```python
from build123d import *

# Parameters (mm, degrees)
SKETCH1_R           = 10
BOSS_EXTRUDE1_DEPTH = 15.1
SKETCH2_R           = 8.25
CUT_EXTRUDE1_DEPTH  = 7
SKETCH3_R           = 6.35
CUT_EXTRUDE2_DEPTH  = 8.1
SKETCH7_R           = 10
BOSS_EXTRUDE2_DEPTH = 10
BOSS_EXTRUDE2_TAPER = 27
SKETCH8_R           = 5.5
CUT_EXTRUDE3_DEPTH  = 10


with BuildPart() as part:
    # Sketch1 → Boss-Extrude1 (new body)
    with BuildSketch(Plane(origin=(0, 0, 0), x_dir=(1, 0, 0), z_dir=(0, 1, 0))):
        with Locations(Location((0, 0, 0), (0, 0, 270))):
            Circle(SKETCH1_R)
    extrude(amount=BOSS_EXTRUDE1_DEPTH)

    # Sketch2 → Cut-Extrude1 (cut)
    with BuildSketch(Plane(origin=(0, 0, 0), x_dir=(-1, 0, 0), z_dir=(0, -1, 0))):
        with Locations(Location((0, 0, 0), (0, 0, 90))):
            Circle(SKETCH2_R)
    extrude(amount=-CUT_EXTRUDE1_DEPTH, mode=Mode.SUBTRACT)

    # Sketch3 → Cut-Extrude2 (cut)
    with BuildSketch(Plane.XZ.offset(-7)):
        with Locations(Location((0, 0, 0), (0, 0, 270))):
            Circle(SKETCH3_R)
    extrude(amount=-CUT_EXTRUDE2_DEPTH, mode=Mode.SUBTRACT)

    # Sketch7 → Boss-Extrude2 (add)
    with BuildSketch(Plane(origin=(0, 15.1, 0), x_dir=(1, 0, 0), z_dir=(0, 1, 0))):
        with Locations(Location((0, 0, 0), (0, 0, 270))):
            Circle(SKETCH7_R)
    extrude(amount=BOSS_EXTRUDE2_DEPTH, taper=BOSS_EXTRUDE2_TAPER)

    # Sketch8 → Cut-Extrude3 (cut)
    with BuildSketch(Plane(origin=(0, 25.1, 0), x_dir=(1, 0, 0), z_dir=(0, 1, 0))):
        with Locations(Location((0, 0, 0), (0, 0, 270))):
            Circle(SKETCH8_R)
    extrude(amount=-CUT_EXTRUDE3_DEPTH, mode=Mode.SUBTRACT)

    # Sketch9 → Cut-Revolve1 (revolve, cut)
    with BuildSketch(Plane.XY, mode=Mode.PRIVATE) as cut_revolve1_sk:
        Polygon((10, 0), (10, 7.55), (9, 0), align=None)
    revolve(cut_revolve1_sk.sketch.rotate(Axis((0, -5.35411367, 0), (0, 1, 0)), 90), axis=Axis((0, -5.35411367, 0), (0, 1, 0)), mode=Mode.SUBTRACT)


solid = part.part
```
Geometry: final body of the model. Coordinates: model frame, mm. A direction names the side the tool comes from. Round coordinates to 2 decimals unless told otherwise and drop trailing zeros. Loops run counter-clockwise (first coordinate to the right, second up) from the corner with the lowest first, then second, coordinate; pieces in that order, holes last. Notation, with made-up numbers: (70.25, 34.25) -> (115.25, 34.25) arc R20 cw to (115.25, 68.25) -> close; hole circle Ø3 at (66, 22). An arc over 180 degrees is marked (long way). Use one line per item in the form item = value.
Item 1: Material intervals for probe 1 along X at (y, z) = (9, 0); probe 2 along X at (y, z) = (3, 0); probe 3 along Z at (x, y) = (1, 22.25), sorted ascending.
Evaluation:
probe_1 = -10 to -6.35, 6.35 to 10
probe_2 = -9.4 to -8.25, 8.25 to 9.4
probe_3 = -6.28 to -5.41, 5.41 to 6.28
Item 2: Cut plane B-B on y = 11. Output: boundary loops of the cut face in (x, z), then the cut area to 3 significant figures.
Evaluation:
outline = circle Ø20 at (0, 0); hole circle Ø12.7 at (0, 0)
area = 187 mm2
Item 3: Contact query for flat-ended pins moving along their axis: pin 1 Ø6 at (x, z) = (0.5, 3) entering from +Y; pin 2 Ø8 at (x, y) = (5.5, 9.5) entering from +Z; pin 3 Ø5 at (x, z) = (4, -0.5) entering from -Y; pin 4 Ø1 at (x, z) = (7, -7.5) entering from +Y. Output: stop coordinate, or through.
Evaluation:
pin_1 = 23.93
pin_2 = 9.89
pin_3 = 7
pin_4 = 15.57
Item 4: Cut plane A-A on z = 0. Output: boundary loops of the cut face in (x, y).
Evaluation:
outline = (-10, 7.55) -> (-9, 0) -> (-8.25, 0) -> (-8.25, 7) -> (-6.35, 7) -> (-6.35, 15.1) -> (-5.5, 15.1) -> (-5.5, 23.93) -> (-10, 15.1) -> close; (5.5, 15.1) -> (6.35, 15.1) -> (6.35, 7) -> (8.25, 7) -> (8.25, 0) -> (9, 0) -> (10, 7.55) -> (10, 15.1) -> (5.5, 23.93) -> close
Item 5: Cut plane C-C on y = 19.25. Output: boundary loops of the cut face in (x, z), then the cut area to 3 significant figures.
Evaluation:
outline = circle Ø15.77 at (0, 0); hole circle Ø11 at (0, 0)
area = 100 mm2
Item 6: Access query for faces 5 (the conical face through (-3.784, 22.522, -4.935)), 6 (the cylindrical face through (-8.054, 3.451, 1.788)). Directions: +Z, -Z, +X, -X, +Y, -Y. A direction counts if a zero-diameter tool reaches every point of the face in a straight line with its end or side. Return the directions, or none.
Evaluation:
face_5 = +Y
face_6 = -Y
Item 7: Draft query along X for faces 1 (the cylindrical face through (-5.37, 19.58, -1.19)), 2 (the flat face through (-6.1, 7, -2.4)), 3 (the flat face through (-3, 0, 8)), 4 (the cylindrical face through (-9.76, 11.27, -2.17)). Return one class per face: released by +X, released by -X, zero draft, split by the parting line, or undercut.
Evaluation:
face_1 = undercut
face_2 = undercut
face_3 = zero draft
face_4 = split by the parting line
